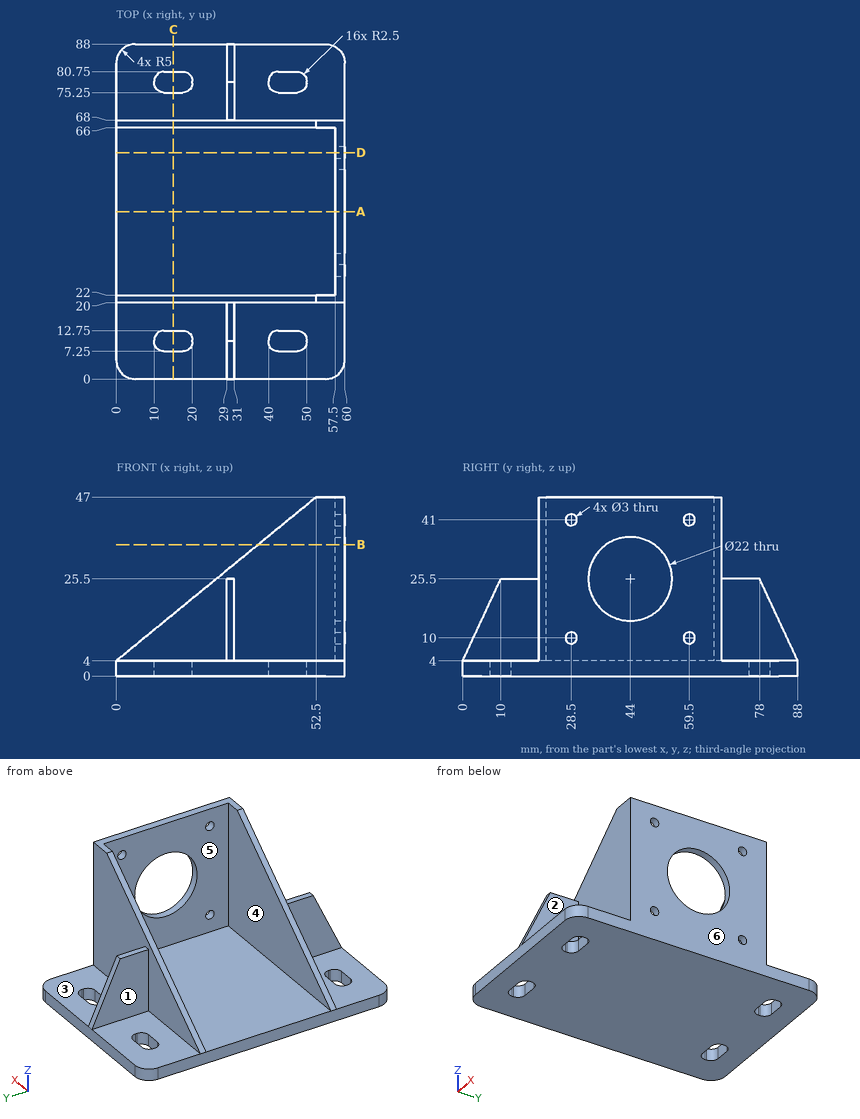
Check sheet for the drawn part. Datum: minimum x, y, z corner. Units: mm. A direction names the side the tool comes from. Round coordinates to 2 decimals unless told otherwise and drop trailing zeros. Order: outer loops, then holes, each group sorted by start corner. A loop starts at its lowest first (then second) coordinate and runs counter-clockwise, first axis right, second up. Notation, with made-up numbers: M -35.75,50.25 L -7.75,50.25 A17 cw -7.75,58.25 Z; hole C 87,30.5 d3. An arc over 180 degrees is marked long. Write each question's results on one line, items separated by ' | '. Start each with the question number.
1. Cross-section at C-C on x = 15. Record the boundary of the cut face in (y, z), plus the area to 3 significant figures.
2. Draft check along Y on the marked faces 5 and 6. Enter one of: pulls with the +Y half, pulls with the -Y half, needs draft (parallel to the pull), parting line crosses it, or undercut.
3. Set-up check for the marked faces 1, 2, 3 and 4: record each of +Z, -Z, +X, -X, +Y, -Y from which the full face is reachable in a straight line by a thin tool's end or side.
4. Cross-section at A-A on y = 44. Record the boundary of the cut face in (x, z).
5. Cross-section at D-D on y = 59.5. Record the boundary of the cut face in (x, z).
6. Go/stop test with flat-tipped pins: P1, Ø1, axis at y = 68, z = 15, coming from the -X side; P2, Ø4, axis at y = 63, z = 25.5, coming from the -X side; P3, Ø21.5, axis at x = 29.5, z = 32, coming from the +Y side. Record where each tip stops, or that it passes through.
7. Material ranges on L1, parallel to Z at x = 58.55, y = 59.5; L2, parallel to Y at x = 56, z = 13.5; L3, parallel to Z at x = 58, y = 44, recorded low to high. Write a range as from..to.
8. Cross-section at B-B on z = 34.5. Record the boundary of the cut face in (x, y).
Resolved:
1) outline: M 0,0 L 7.25,0 L 7.25,4 L 0,4 Z; M 12.75,0 L 75.25,0 L 75.25,4 L 68,4 L 68,16.29 L 66,16.29 L 66,4 L 22,4 L 22,16.29 L 20,16.29 L 20,4 L 12.75,4 Z; M 80.75,0 L 88,0 L 88,4 L 80.75,4 Z | area: 357 mm2
2) face 5: undercut | face 6: needs draft
3) face 1: +Z, -X, +Y | face 2: +Z, +X, -Y | face 3: +Z, +X, +Y | face 4: +Z, -X
4) outline: M 0,0 L 60,0 L 60,14.5 L 57.5,14.5 L 57.5,4 L 0,4 Z; M 57.5,36.5 L 60,36.5 L 60,47 L 57.5,47 Z
5) outline: M 0,0 L 60,0 L 60,8.5 L 57.5,8.5 L 57.5,4 L 0,4 Z; M 57.5,11.5 L 60,11.5 L 60,39.5 L 57.5,39.5 Z; M 57.5,42.5 L 60,42.5 L 60,47 L 57.5,47 Z
6) P1: x = 12.82 | P2: x = 57.5 | P3: y = 79.98
7) L1: 0..8.5, 11.5..39.5, 42.5..47 | L2: 20..22, 66..68 | L3: 0..14.5, 36.5..47
8) outline: M 37.24,20 L 60,20 L 60,37.68 L 57.5,37.68 L 57.5,22 L 37.24,22 Z; M 37.24,66 L 57.5,66 L 57.5,50.32 L 60,50.32 L 60,68 L 37.24,68 Z
